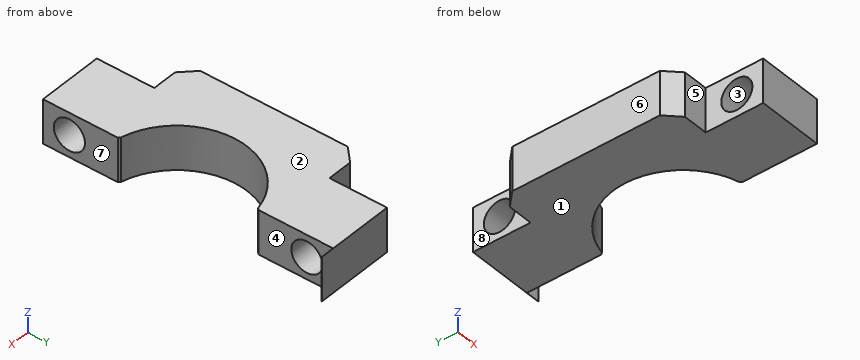
from build123d import *

# Parameters (mm, degrees)
BOSS_EXTRUDE2_DEPTH  = 3.175
CHAMFER2_SIZE        = 2
M4_CLEARANCE_HOLE1_D = 4.5
CHAMFER1_SIZE        = 2
SKETCH6_W            = 2
SKETCH6_H            = 41.891167458
CUT_EXTRUDE1_DEPTH   = 28.75134276


with BuildPart() as part:
    # Sketch1 → Boss-Extrude2 (new, symmetric)
    with BuildSketch(Plane.XY):
        with BuildLine():
            Line((0, 10.16), (0, 20.955))
            Line((0, 20.955), (-11.43, 20.955))
            Line((-11.43, 20.955), (-11.43, 12.651387276))
            Line((-11.43, 12.651387276), (-17.05, 12.651387276))
            Line((-17.05, 12.651387276), (-17.05, -12.651387276))
            Line((-17.05, -12.651387276), (-11.43, -12.651387276))
            Line((-11.43, -12.651387276), (-11.43, -20.955))
            Line((-11.43, -20.955), (0, -20.955))
            Line((0, -20.955), (0, -10.16))
            ThreePointArc((0, -10.16), (-10.16, 0), (0, 10.16))
        make_face()
    extrude(amount=BOSS_EXTRUDE2_DEPTH, both=True)

    # Chamfer2
    chamfer2_edges = [part.edges().sort_by_distance(p)[0] for p in [
        (-17.05, -12.651387276, 0),
        (-17.05, 12.651387276, 0),
    ]]
    chamfer(chamfer2_edges, length=CHAMFER2_SIZE)

    # M4 Clearance Hole1 (through all)
    with Locations(Plane.ZY.offset(17.05)):
        with Locations((0, 17.145), (0, -17.145)):
            Hole(M4_CLEARANCE_HOLE1_D / 2)

    # Chamfer1
    # the kernel refuses this chamfer: 2 mm, written as the material it takes off along each edge
    with BuildSketch(Plane(origin=(0, -10.16, 9.000384751), x_dir=(-0.9937566306409056, 0.1115695256655456, 0), z_dir=(0, 0, -1))) as chamfer1_piece_1:
        with BuildLine():
            Line((2.267092762, 0), (-CHAMFER1_SIZE * 0.111569525666, -CHAMFER1_SIZE * 0.993756630641))
            Line((-CHAMFER1_SIZE * 0.111569525666, -CHAMFER1_SIZE * 0.993756630641), (0, 0))
            ThreePointArc((0, 0), (1.165083929, -0.063383685), (2.267092762, 0))
        make_face()
    extrude(amount=18.000769503, mode=Mode.SUBTRACT)
    with BuildSketch(Plane(origin=(0, 10.16, 9.000384751), x_dir=(0, 1, 0), z_dir=(0, 0, -1))) as chamfer1_piece_2:
        with BuildLine():
            Line((CHAMFER1_SIZE, 0), (-0.252938464, -2.252938464))
            ThreePointArc((-0.252938464, -2.252938464), (-0.066999904, -1.164881567), (0, 0))
            Line((0, 0), (CHAMFER1_SIZE, 0))
        make_face()
    extrude(amount=18.000769503, mode=Mode.SUBTRACT)

    # Sketch6 → Cut-Extrude1 (cut, through all)
    with BuildSketch(Plane.XY.offset(3.175)):
        with Locations((-1, -0.009416271)):
            Rectangle(SKETCH6_W, SKETCH6_H)
    extrude(amount=-CUT_EXTRUDE1_DEPTH, mode=Mode.SUBTRACT)


solid = part.part
Source: CAD feature listing. Evaluate the final solid. Frame: model axes, mm. Face numbers are marked on the shaded views. A direction names the side the tool comes from. Coordinates: 2 decimals unless noted, no trailing zeros. Order: outer loops, then holes, each group sorted by start corner. A loop starts at its lowest first (then second) coordinate and runs counter-clockwise, first axis right, second up. Notation, with made-up numbers: M 81.5,22.25 L 86.5,22.25 A24 cw 86.5,48.25 Z; hole C -27,-36.5 d5. An arc over 180 degrees is marked long. Write each question's results on one line, items separated by ' | '. Start each with the question number.
1. Material intervals for L1, parallel to Y at x = -2.25, z = -1.75 (3 decimals); L2, parallel to Y at x = -5, z = 0 (3 decimals); L3, parallel to Y at x = -12, z = -2, sorted ascending.
2. Section C-C, the plane y = -16. Return the cut outline in (x, z) (3 decimals).
3. Draft query along Z for the marked faces 1, 2, 3 and 4. Return one class per face: +Z half, -Z half, draft (parallel to the pull), parting line (faces both ways), or undercut.
4. Section A-A, the plane z = 0. Return the cut outline in (x, y) (3 decimals).
5. Pin query (flat end, axial travel): pin 1 (3 mm diameter, centred on x = -13, y = 16, fed in from -Z); pin 2 (2 mm diameter, centred on y = 0, z = -1, fed in from +X); pin 3 (3 mm diameter, centred on y = -16.5, z = -0.5, fed in from +X). Return the tip coordinate at first contact, or that it passes through.
6. Reachability of the marked faces 5, 6, 7 and 8 from +Z, -Z, +X, -X, +Y, -Y: full face, straight path, thin tool, end or side. Return the list, or none.
7. Section B-B, the plane x = -8.75. Return the cut outline in (y, z) (3 decimals), then the cut area to 3 significant figures.
8. Section D-D, the plane x = -12.75. Return the cut outline in (y, z) (3 decimals).
Solution:
1) L1: -20.955 to -18.559, -15.731 to -9.91, 9.91 to 15.731, 18.559 to 20.955 | L2: -20.955 to -19.395, -14.895 to -8.845, 8.845 to 14.895, 19.395 to 20.955 | L3: -12.65 to 12.65
2) outline: M -11.43,-3.175 L -2,-3.175 L -2,-1.937 L -11.43,-1.937 Z; M -11.43,1.937 L -2,1.937 L -2,3.175 L -11.43,3.175 Z
3) face 1: -Z half | face 2: +Z half | face 3: undercut | face 4: draft
4) outline: M -17.05,-10.651 L -15.05,-12.651 L -11.43,-12.651 L -11.43,-14.895 L -2,-14.895 L -2,-10.16 L -2.253,-9.907 A10.16 cw -2.253,9.907 L -2,10.16 L -2,14.895 L -11.43,14.895 L -11.43,12.651 L -15.05,12.651 L -17.05,10.651 Z; M -11.43,-20.955 L -2,-20.955 L -2,-19.395 L -11.43,-19.395 Z; M -11.43,19.395 L -2,19.395 L -2,20.936 L 0,20.936 L 0,20.955 L -11.43,20.955 Z
5) pin 1: through | pin 2: x = -10.11 | pin 3: x = -2
6) face 5: +Z, -Z, -X, -Y | face 6: +Z, -Z, -X, +Y, -Y | face 7: +Z, -Z, +X, -Y | face 8: +Z, -Z, -X, +Y
7) outline: M -20.955,-3.175 L -5.164,-3.175 L -5.164,3.175 L -20.955,3.175 Z; M 5.164,-3.175 L 20.955,-3.175 L 20.955,3.175 L 5.164,3.175 Z; hole C -17.145,0 d4.5; hole C 17.145,0 d4.5 | area: 169 mm²
8) outline: M -12.651,-3.175 L 12.651,-3.175 L 12.651,3.175 L -12.651,3.175 Z
